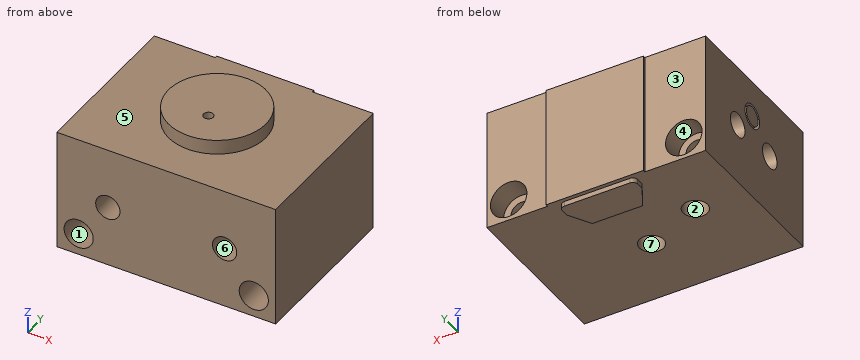
from build123d import *

# Parameters (mm, degrees)
SKETCH1_W                     = 45
SKETCH1_H                     = 33.5
BASE_EXTRUDE_DEPTH            = 25
SKETCH2_W                     = 20
SKETCH2_H                     = 0.5
TOPBOSS_DEPTH                 = 25
SKETCH3_R                     = 10
INSERT_DEPTH                  = 3
SKETCH5_R                     = 3.75
TOPCBORES_DEPTH               = 4.5
SKETCH6_R                     = 2.25
TOPTHRUHOLES_DEPTH            = 47.165463282
PORTTHRUHOLETOP_DEPTH         = 40.956226048
PORTTHRUHOLETOP_DEPTH_BACK    = 40.956226048
SKETCH18_R                    = 1
SKETCH24_R                    = 1
PORTTHRUHOLEBOTTOM_DEPTH      = 56.814424659
SKETCH25_R                    = 2.5
SIDEACBORETOP_DEPTH           = 5
SIDEBCBORETOP_START           = -5
SKETCH26_R                    = 2.5
SIDEBCBORETOP_DEPTH           = 5
SKETCH28_R                    = 2.5
SIDEACBOREBOTTOM_DEPTH        = 5
SIDEBCBOREBOTTOM_START        = -5
SKETCH29_R                    = 2.5
SIDEBCBOREBOTTOM_DEPTH        = 5
SKETCH19_R                    = 2.5
CVALVECUT2_DEPTH              = 2
SKETCH30_R                    = 2
CVALVE2_DEPTH                 = 2
SKETCH20_R                    = 2.5
EXTRUDE_1_DEPTH               = 4
SKETCH21_R                    = 2.5
EXTRUDE_2_DEPTH               = 4
SKETCH35_R                    = 2.5
CENTERENDPORTH_R_G_DEPTH      = 5
SKETCH36_R                    = 1
CENTERENDPORTH_R_G_THRU_DEPTH = 37.626493144
SKETCH37_R                    = 2.5
OFFCENTERENDPORTH_R_DEPTH     = 5
SKETCH38_R                    = 1
OFFCENTERENDPORTH_RTHRU_DEPTH = 5
PLASTICCAP_DEPTH              = 1
SKETCH40_R                    = 2.5
BOTTOMPORTS_DEPTH             = 5
SKETCH41_R                    = 1
BOTTOMAPASSAGE_DEPTH          = 22.5
SKETCH42_R                    = 1
BOTTOMBPASSAGE_DEPTH          = 11.5
SKETCH43_R                    = 3
CUT_EXTRUDE1_DEPTH            = 12


with BuildPart() as part:
    # Sketch1 → Base-Extrude (new body)
    with BuildSketch(Plane.XY):
        with Locations((0, -0.75)):
            Rectangle(SKETCH1_W, SKETCH1_H)
    extrude(amount=BASE_EXTRUDE_DEPTH)

    # Sketch2 → TopBoss (add)
    with BuildSketch(Plane.XY):
        with Locations((0, 16.25)):
            Rectangle(SKETCH2_W, SKETCH2_H)
    extrude(amount=TOPBOSS_DEPTH)

    # Sketch3 → Insert (add)
    with BuildSketch(Plane.XY.offset(25)):
        Circle(SKETCH3_R)
    extrude(amount=INSERT_DEPTH)

    # Sketch5 → TopCbores (cut)
    with BuildSketch(Plane(origin=(0, 16, 0), x_dir=(-1, 0, 0), z_dir=(0, 1, 0))):
        with Locations(Location((18, 4.5, 0), (0, 0, 90))):
            Circle(SKETCH5_R)
        with Locations(Location((-18, 4.5, 0), (0, 0, 270))):
            Circle(SKETCH5_R)
    extrude(amount=-TOPCBORES_DEPTH, mode=Mode.SUBTRACT)

    # Sketch6 → TopThruHoles (cut, through all)
    with BuildSketch(Plane(origin=(0, 11.5, 0), x_dir=(-1, 0, 0), z_dir=(0, 1, 0))):
        with Locations(Location((-18, 4.5, 0), (0, 0, 90))):
            Circle(SKETCH6_R)
        with Locations(Location((18, 4.5, 0), (0, 0, 90))):
            Circle(SKETCH6_R)
    extrude(amount=-TOPTHRUHOLES_DEPTH, mode=Mode.SUBTRACT)

    # Sketch18 → PortThruHoleTop (cut, two sides: drawn at the far end of the back side and taken through both)
    with BuildSketch(Plane(origin=(0, 0, 0), x_dir=(0, 0, -1), z_dir=(1, 0, 0)).offset(-PORTTHRUHOLETOP_DEPTH_BACK)):
        with Locations((-12.5, 5)):
            Circle(SKETCH18_R)
    extrude(amount=PORTTHRUHOLETOP_DEPTH + PORTTHRUHOLETOP_DEPTH_BACK, mode=Mode.SUBTRACT)

    # Sketch24 → PortThruHoleBottom (cut, through all)
    with BuildSketch(Plane(origin=(22.5, 0, 0), x_dir=(0, 0, -1), z_dir=(1, 0, 0))):
        with Locations(Location((-12.5, -6, 0), (0, 0, 90))):
            Circle(SKETCH24_R)
    extrude(amount=-PORTTHRUHOLEBOTTOM_DEPTH, mode=Mode.SUBTRACT)

    # Sketch25 → SideACboreTop (cut)
    with BuildSketch(Plane(origin=(22.5, 0, 0), x_dir=(0, 0, -1), z_dir=(1, 0, 0))):
        with Locations(Location((-12.5, 5, 0), (0, 0, 90))):
            Circle(SKETCH25_R)
    extrude(amount=-SIDEACBORETOP_DEPTH, mode=Mode.SUBTRACT)

    # Sketch26 → SideBCboreTop (cut)
    with BuildSketch(Plane.ZY.offset(22.5).offset(SIDEBCBORETOP_START)):
        with Locations(Location((12.5, 5, 0), (0, 0, 90))):
            Circle(SKETCH26_R)
    extrude(amount=SIDEBCBORETOP_DEPTH, mode=Mode.SUBTRACT)

    # Sketch28 → SideACboreBottom (cut)
    with BuildSketch(Plane(origin=(22.5, 0, 0), x_dir=(0, 0, -1), z_dir=(1, 0, 0))):
        with Locations(Location((-12.5, -6, 0), (0, 0, 90))):
            Circle(SKETCH28_R)
    extrude(amount=-SIDEACBOREBOTTOM_DEPTH, mode=Mode.SUBTRACT)

    # Sketch29 → SideBCboreBottom (cut)
    with BuildSketch(Plane.ZY.offset(22.5).offset(SIDEBCBOREBOTTOM_START)):
        with Locations(Location((12.5, -6, 0), (0, 0, 90))):
            Circle(SKETCH29_R)
    extrude(amount=SIDEBCBOREBOTTOM_DEPTH, mode=Mode.SUBTRACT)

    # Sketch19 → CValveCut2 (cut)
    with BuildSketch(Plane.ZY.offset(22.5)):
        with Locations(Location((17.5, 0, 0), (0, 0, 270))):
            Circle(SKETCH19_R)
    extrude(amount=-CVALVECUT2_DEPTH, mode=Mode.SUBTRACT)

    # Sketch30 → CValve2 (add)
    with BuildSketch(Plane.ZY.offset(20.5)):
        with Locations(Location((17.5, 0, 0), (0, 0, 90))):
            Circle(SKETCH30_R)
    extrude(amount=CVALVE2_DEPTH)

    # Sketch20 → 1 (add)
    with BuildSketch(Plane(origin=(22.5, 0, 0), x_dir=(0, 0, -1), z_dir=(1, 0, 0))):
        with Locations(Location((-12.5, 5, 0), (0, 0, 90))):
            Circle(SKETCH20_R)
    extrude(amount=-EXTRUDE_1_DEPTH)

    # Sketch21 → 2 (add)
    with BuildSketch(Plane(origin=(22.5, 0, 0), x_dir=(0, 0, -1), z_dir=(1, 0, 0))):
        with Locations(Location((-12.5, -6, 0), (0, 0, 90))):
            Circle(SKETCH21_R)
    extrude(amount=-EXTRUDE_2_DEPTH)

    # Sketch35 → CenterEndPortH&R_G (cut)
    with BuildSketch(Plane(origin=(0, 0, 0), x_dir=(-1, 0, 0), z_dir=(0, 0, -1))):
        with Locations((0, -3)):
            Circle(SKETCH35_R)
    extrude(amount=-CENTERENDPORTH_R_G_DEPTH, mode=Mode.SUBTRACT)

    # Sketch36 → CenterEndPortH&R_G_Thru (cut, through all)
    with BuildSketch(Plane(origin=(0, 0, 5), x_dir=(-1, 0, 0), z_dir=(0, 0, -1))):
        with Locations((0, -3)):
            Circle(SKETCH36_R)
    extrude(amount=-CENTERENDPORTH_R_G_THRU_DEPTH, mode=Mode.SUBTRACT)

    # Sketch37 → OffCenterEndPortH&R (cut)
    with BuildSketch(Plane(origin=(0, 0, 0), x_dir=(-1, 0, 0), z_dir=(0, 0, -1))):
        with Locations((12, 2)):
            Circle(SKETCH37_R)
    extrude(amount=-OFFCENTERENDPORTH_R_DEPTH, mode=Mode.SUBTRACT)

    # Sketch38 → OffCenterEndPortH&RThru (cut)
    with BuildSketch(Plane(origin=(0, 0, 5), x_dir=(-1, 0, 0), z_dir=(0, 0, -1))):
        with Locations((12, 2)):
            Circle(SKETCH38_R)
    extrude(amount=-OFFCENTERENDPORTH_RTHRU_DEPTH, mode=Mode.SUBTRACT)

    # Sketch39 → PlasticCap (add)
    with BuildSketch(Plane(origin=(0, 0, 0), x_dir=(-1, 0, 0), z_dir=(0, 0, -1))):
        with BuildLine():
            Line((-6.75, 15.7), (6.75, 15.7))
            ThreePointArc((6.75, 15.7), (7.457106781, 15.407106781), (7.75, 14.7))
            Line((7.75, 14.7), (7.75, 13.2))
            Line((7.75, 13.2), (5.151923789, 8.7))
            Line((5.151923789, 8.7), (-5.151923789, 8.7))
            Line((-5.151923789, 8.7), (-7.75, 13.2))
            Line((-7.75, 13.2), (-7.75, 14.7))
            ThreePointArc((-7.75, 14.7), (-7.457106781, 15.407106781), (-6.75, 15.7))
        make_face()
    extrude(amount=PLASTICCAP_DEPTH)

    # Sketch40 → BottomPorts (cut)
    with BuildSketch(Plane.XZ.offset(17.5)):
        with Locations(Location((12, 12.5, 0), (0, 0, 270))):
            Circle(SKETCH40_R)
        with Locations(Location((-12, 12.5, 0), (0, 0, 270))):
            Circle(SKETCH40_R)
    extrude(amount=-BOTTOMPORTS_DEPTH, mode=Mode.SUBTRACT)

    # Sketch41 → BottomAPassage (cut)
    with BuildSketch(Plane.XZ.offset(17.5)):
        with Locations(Location((12, 12.5, 0), (0, 0, 270))):
            Circle(SKETCH41_R)
    extrude(amount=-BOTTOMAPASSAGE_DEPTH, mode=Mode.SUBTRACT)

    # Sketch42 → BottomBPassage (cut)
    with BuildSketch(Plane.XZ.offset(17.5)):
        with Locations(Location((-12, 12.5, 0), (0, 0, 270))):
            Circle(SKETCH42_R)
    extrude(amount=-BOTTOMBPASSAGE_DEPTH, mode=Mode.SUBTRACT)

    # Sketch43 → Cut-Extrude1 (cut)
    with BuildSketch(Plane.XZ.offset(17.5)):
        with Locations((-18, 4.5)):
            Circle(SKETCH43_R)
        with Locations((18, 4.5)):
            Circle(SKETCH43_R)
    extrude(amount=-CUT_EXTRUDE1_DEPTH, mode=Mode.SUBTRACT)


solid = part.part
The listing builds one solid part. Answer for the finished solid, in the listing's coordinates (mm). Face numbers are marked on the shaded views. A direction names the side the tool comes from. Give positions to 0.01 mm unless a question says otherwise; leave off trailing zeros. Write each loop counter-clockwise with the first axis right and the second up, starting at its lowest first coordinate (ties: lowest second). Pieces come first, ordered by that corner, then holes.
Item 1: Section B-B, the plane x = -12 is taken. Write down the section's boundary in (y, z).
Item 2: Which of the six approach directions +Z, -Z, +X, -X, +Y, -Y give full straight-line access (tool end or side, diameter ignored) to the marked faces 4, 5, 6 and 7?
Item 3: Determine the mould class of the marked faces 1, 2 and 3 for opening direction Y: released by +Y, released by -Y, zero draft, split by the parting line, or undercut.
Item 4: Flat-ended cylindrical pins translate along their axes: P1, Ø6, axis at x = -18, z = 5.5, coming from the +Y side; P2, Ø5.5, axis at x = -12.5, y = 3, coming from the -Z side; P3, Ø0.5, axis at x = -3.5, z = -0.5, coming from the +Y side. Find the tip coordinate at first contact, or state that the pin passes through.
Item 5: Section A-A, the plane x = 0 is taken. Write down the section's boundary in (y, z).
Item 6: Find the intervals of material crossed by line 1 along Y through (x, z) = (-6, 12.5); line 2 along X through (y, z) = (-15.35, 12.5); line 3 along Z through (x, y) = (-11.5, -6), in increasing order.
Completed:
1. outline: (-17.5, 0) - (-0.5, 0) - (-0.5, 5) - (1, 5) - (1, 10) - (3, 10) - (3, 5) - (4.5, 5) - (4.5, 0) - (16, 0) - (16, 25) - (-17.5, 25) - (-17.5, 15) - (-12.5, 15) - (-12.5, 13.5) - (-6, 13.5) arc R1 cw to (-6, 11.5) - (-12.5, 11.5) - (-12.5, 10) - (-17.5, 10) - close; hole circle Ø2 at (5, 12.5)
2. face 4: +Y
2. face 5: +Z
2. face 6: -Y
2. face 7: -Z
3. face 1: zero draft
3. face 2: undercut
3. face 3: released by +Y
4. P1: stops at y = 16
4. P2: stops at z = 0
4. P3: stops at y = 15.7
5. outline: (-17.5, 0) - (-5.5, 0) - (-5.5, 5) - (-4, 5) - (-4, 28) - (-10, 28) - (-10, 25) - (-17.5, 25) - close; (-2, 5) - (-0.5, 5) - (-0.5, 0) - (8.7, 0) - (8.7, -1) - (15.7, -1) - (15.7, 0) - (16.5, 0) - (16.5, 25) - (10, 25) - (10, 28) - (-2, 28) - close; hole circle Ø2 at (-6, 12.5); hole circle Ø2 at (5, 12.5)
6. line 1: y = -17.5 to -7, -5 to 4, 6 to 16.5
6. line 2: x = -22.5 to -14.5, -9.5 to 9.5, 14.5 to 22.5
6. line 3: z = 0 to 11.5, 13.5 to 25
